Design review of the part built by this model. Coordinates are the model's own, in mm. Face numbers are marked on the shaded views. Round coordinates to 2 decimals unless told otherwise and drop trailing zeros. Loops run counter-clockwise (first coordinate to the right, second up) from the corner with the lowest first, then second, coordinate; pieces in that order, holes last. Notation, with made-up numbers: (-28.5, -8.75) - (-8.5, -8.75) arc R23 ccw to (-8.5, 5.25) - close; hole circle Ø9 at (41.5, 44). An arc over 180 degrees is marked (long way). Return JSON: item names as keys, results as strings. Group by question number.
(1) We need section D-D, the plane y = 49. Write out the cut boundary in (x, z).
(2) We need section C-C, the plane z = -2.75. Write out the cut boundary in (x, y) (3 decimals), and give its area (3 significant figures).
(3) We need section B-B, the plane x = -1.25. Write out the cut boundary in (y, z), and give its area (3 significant figures).
(4) The part is to be moulded in two halves that separate along X. For the marked faces 1, 2, 3 and 4, say which applies: pulls with the +X half, pulls with the -X half, needs draft (parallel to the pull), parting line crosses it, or undercut.
(5) We need section A-A, the plane x = 1.5. Write out the cut boundary in (y, z).
(6) Wall thickness on L1, parallel to Y at x = 0, z = 0.65; L2, parallel to X at y = 2.5, z = 2.5 (3 decimals); L3, parallel to X at y = 35.5, z = 1.75: over which ranges is each line inside the solid? List them lowest first. Write a range as [from, to].
(7) Clearance check with flat-ended pins moving along their axes: pin 1 (0.6 mm diameter, centred on x = 0, z = 2, fed in from -Y); pin 2 (4 mm diameter, centred on x = 3.5, z = -3, fed in from -Y); pin 3 (1.5 mm diameter, centred on y = 4.01, z = -2.5, fed in from +X); pin 4 (6.5 mm diameter, centred on x = 3, y = 28.5, fed in from +Z). State where each tip first meets the part, or that it passes through.
from build123d import *

# Parameters (mm, degrees)
EXTRUDE_1_DEPTH          = 4
CUT_EXTRUDE_1_DEPTH      = 3
SKETCH_4_R               = 2.6
CUT_EXTRUDE_9_DEPTH      = 19
CUT_EXTRUDE_9_DEPTH_BACK = 2
SKETCH_5_W               = 0.75
SKETCH_5_H               = 13
CUT_EXTRUDE_11_DEPTH     = 5
SKETCH_8_W               = 5
SKETCH_8_H               = 5
EXTRUDE_2_DEPTH          = 5
SKETCH_9_R               = 1.25
CUT_EXTRUDE_12_DEPTH     = 39
SKETCH_11_W              = 5
SKETCH_11_H              = 3.5
SKETCH_11_R              = 1.25
EXTRUDE_4_DEPTH          = 5


with BuildPart() as part:
    # 草圖1 → 填料-伸長1 (new body)
    with BuildSketch(Plane.XY):
        with BuildLine():
            Line((-9, 0), (-9, 50))
            ThreePointArc((-9, 50), (0, 59), (9, 50))
            Line((9, 50), (9, 0))
            Line((9, 0), (-9, 0))
        make_face()
    extrude(amount=EXTRUDE_1_DEPTH)

    # 草圖2 → 除料-伸長1 (cut)
    with BuildSketch(Plane.XY.offset(4)):
        with BuildLine():
            Line((-2.6, 53.145110573), (-5, 39.352358854))
            ThreePointArc((-5, 39.352358854), (-6.5, 35.199046922), (-5, 31.045734991))
            Line((-5, 31.045734991), (-2.656326538, 17.243300615))
            ThreePointArc((-2.656326538, 17.243300615), (0, 15), (2.656326538, 17.243300615))
            Line((2.656326538, 17.243300615), (5, 31.045734991))
            ThreePointArc((5, 31.045734991), (6.5, 35.199046922), (5, 39.352358854))
            Line((5, 39.352358854), (2.6, 53.145110573))
            ThreePointArc((2.6, 53.145110573), (0, 55.331766334), (-2.6, 53.145110573))
        make_face()
    extrude(amount=-CUT_EXTRUDE_1_DEPTH, mode=Mode.SUBTRACT)

    # 草圖4 → 除料-伸長9 (cut, two sides)
    with BuildSketch(Plane.XY) as cut_extrude_9_sk:
        with Locations((0, 34.856314216)):
            Circle(SKETCH_4_R)
    extrude(amount=CUT_EXTRUDE_9_DEPTH, mode=Mode.SUBTRACT)
    extrude(cut_extrude_9_sk.sketch, amount=-CUT_EXTRUDE_9_DEPTH_BACK, mode=Mode.SUBTRACT)

    # 草圖5 → 除料-伸長11 (cut, through all)
    with BuildSketch(Plane.XY):
        with Locations((0, 6.5)):
            Rectangle(SKETCH_5_W, SKETCH_5_H)
    extrude(amount=CUT_EXTRUDE_11_DEPTH, mode=Mode.SUBTRACT)

    # 草圖8 → 填料-伸長2 (add)
    with BuildSketch(Plane.XY):
        with Locations((2.875, 8.312164066)):
            Rectangle(SKETCH_8_W, SKETCH_8_H)
    extrude(amount=-EXTRUDE_2_DEPTH)

    # 草圖9 → 除料-伸長12 (cut)
    with BuildSketch(Plane(origin=(0, 0, 0), x_dir=(0, 0, -1), z_dir=(1, 0, 0))):
        with Locations((2.379774756, 8.312164066)):
            Circle(SKETCH_9_R)
    extrude(amount=CUT_EXTRUDE_12_DEPTH, mode=Mode.SUBTRACT)

    # 草圖11 → 填料-伸長4 (add)
    with BuildSketch(Plane(origin=(0.375, 0, 0), x_dir=(0, 0, -1), z_dir=(1, 0, 0))):
        with Locations((2.5, 4.012164066)):
            Rectangle(SKETCH_11_W, SKETCH_11_H)
        with Locations((2.5, 4.012164066)):
            Circle(SKETCH_11_R, mode=Mode.SUBTRACT)
    extrude(amount=EXTRUDE_4_DEPTH)


solid = part.part
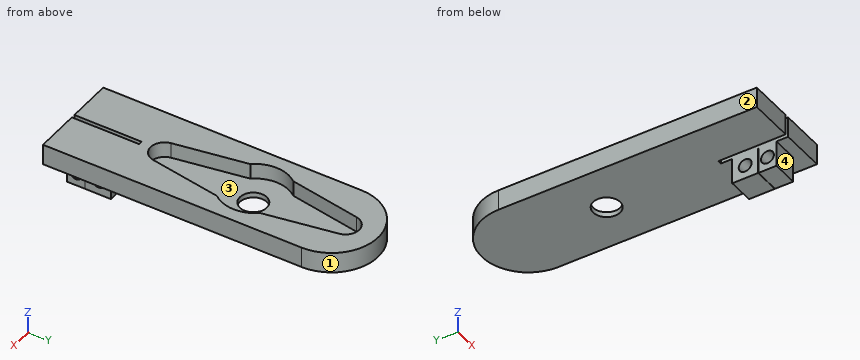
Solutions:
{
 "1": {"outline": "(-9, 0) - (9, 0) - (9, 4) - (3.32, 4) - (3.32, 1) - (-3.32, 1) - (-3.32, 4) - (-9, 4) - close"},
 "2": {"outline": "(0.375, 2.262) - (5.375, 2.262) - (5.375, 2.787) - (0.375, 2.787) - close; (0.375, 5.237) - (5.375, 5.237) - (5.375, 5.762) - (0.375, 5.762) - close; (0.375, 5.812) - (5.375, 5.812) - (5.375, 7.118) - (0.375, 7.118) - close; (0.375, 9.506) - (5.375, 9.506) - (5.375, 10.812) - (0.375, 10.812) - close", "area": "18.3 mm^2"},
 "3": {"outline": "(0, 0) - (32.58, 0) - (32.58, 1) - (15.31, 1) - (15.31, 4) - (0, 4) - close; (37.14, 0) - (58.91, 0) - (58.91, 4) - (55.02, 4) - (55.02, 1) - (37.14, 1) - close", "area": "112 mm^2"},
 "4": {"face 1": "parting line crosses it", "face 2": "pulls with the -X half", "face 3": "undercut", "face 4": "needs draft"},
 "5": {"outline": "(0, 0) - (2.26, 0) - (2.26, -5) - (5.76, -5) - (5.76, 0) - (5.81, 0) - (5.81, -5) - (10.81, -5) - (10.81, 0) - (32.73, 0) - (32.73, 1) - (15.46, 1) - (15.46, 4) - (0, 4) - close; (36.98, 0) - (58.87, 0) - (58.87, 4) - (54.86, 4) - (54.86, 1) - (36.98, 1) - close; hole circle Ø2.5 at (4.01, -2.5); hole circle Ø2.5 at (8.31, -2.38)"},
 "6": {"L1": "[13, 32.26], [37.46, 59]", "L2": "[-9, -0.375], [0.375, 9]", "L3": "[-9, -6.49], [6.49, 9]"},
 "7": {"pin 1": "y = 13", "pin 2": "y = 2.26", "pin 3": "through", "pin 4": "z = 4"}
}
